For this review, take the finished solid that the model builds, in its own axes (mm). Face numbers are marked on the shaded views. Round coordinates to 2 decimals unless told otherwise and drop trailing zeros. Write each loop counter-clockwise with the first axis right and the second up, starting at its lowest first coordinate (ties: lowest second). Pieces come first, ordered by that corner, then holes. Notation, with made-up numbers: (-34.5, -38.5) - (8.5, -38.5) arc R11 ccw to (8.5, -30.5) - close; hole circle Ø8 at (45, 8.5). An arc over 180 degrees is marked (long way). Answer in a Markdown table with one row per item. Add a question column.
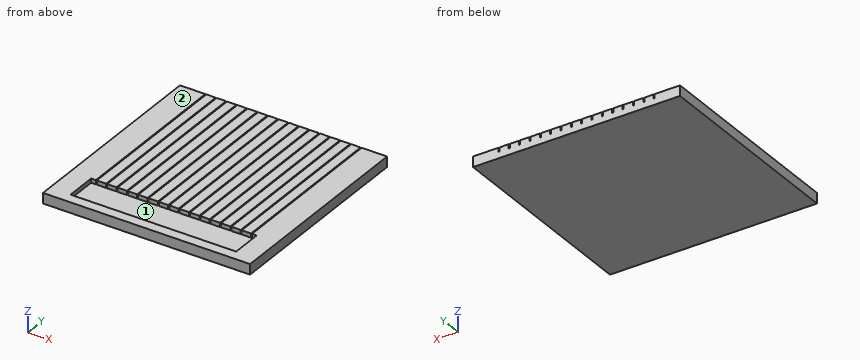
from build123d import *

# Parameters (mm, degrees)
SKETCH1_W           = 10
SKETCH1_H           = 10
BOSS_EXTRUDE1_DEPTH = 0.5
SKETCH2_W           = 8
SKETCH2_H           = 1.5
CUT_EXTRUDE1_DEPTH  = 0.2
SKETCH3_W           = 0.05
SKETCH3_H           = 8
CUT_EXTRUDE2_DEPTH  = 0.2


with BuildPart() as part:
    # Sketch1 → Boss-Extrude1 (new body)
    with BuildSketch(Plane(origin=(0, 0, 0), x_dir=(0, 1, 0), z_dir=(0, 0, 1))):
        with Locations((5, -5)):
            Rectangle(SKETCH1_W, SKETCH1_H)
    extrude(amount=BOSS_EXTRUDE1_DEPTH)

    # Sketch2 → Cut-Extrude1 (cut)
    with BuildSketch(Plane.XY.offset(0.5)):
        with Locations((5, 1.25)):
            Rectangle(SKETCH2_W, SKETCH2_H)
    extrude(amount=-CUT_EXTRUDE1_DEPTH, mode=Mode.SUBTRACT)

    # Sketch3 → Cut-Extrude2 (cut)
    with BuildSketch(Plane.XY.offset(0.5)):
        with Locations((1.25, 6)):
            Rectangle(SKETCH3_W, SKETCH3_H)
        with Locations((1.75, 6)):
            Rectangle(SKETCH3_W, SKETCH3_H)
        with Locations((2.25, 6)):
            Rectangle(SKETCH3_W, SKETCH3_H)
        with Locations((2.75, 6)):
            Rectangle(SKETCH3_W, SKETCH3_H)
        with Locations((3.25, 6)):
            Rectangle(SKETCH3_W, SKETCH3_H)
        with Locations((3.75, 6)):
            Rectangle(SKETCH3_W, SKETCH3_H)
        with Locations((4.25, 6)):
            Rectangle(SKETCH3_W, SKETCH3_H)
        with Locations((4.75, 6)):
            Rectangle(SKETCH3_W, SKETCH3_H)
        with Locations((5.25, 6)):
            Rectangle(SKETCH3_W, SKETCH3_H)
        with Locations((5.75, 6)):
            Rectangle(SKETCH3_W, SKETCH3_H)
        with Locations((6.25, 6)):
            Rectangle(SKETCH3_W, SKETCH3_H)
        with Locations((6.75, 6)):
            Rectangle(SKETCH3_W, SKETCH3_H)
        with Locations((7.25, 6)):
            Rectangle(SKETCH3_W, SKETCH3_H)
        with Locations((7.75, 6)):
            Rectangle(SKETCH3_W, SKETCH3_H)
        with Locations((8.25, 6)):
            Rectangle(SKETCH3_W, SKETCH3_H)
        with Locations((8.75, 6)):
            Rectangle(SKETCH3_W, SKETCH3_H)
    extrude(amount=-CUT_EXTRUDE2_DEPTH, mode=Mode.SUBTRACT)


solid = part.part
Q1. Add section A-A on x = 8.5. State the section outline as (y, z) points.
Q2. Add section B-B on z = 0.4. Count the separate pieces of the cut face and the enclosed holes in it, then the cut area to 3 significant figures.
Q3. Draft analysis for pull direction X (two halves, no side actions). For the marked faces 1 and 2, state which applies: released by +X, released by -X, zero draft, split by the parting line, or undercut.
Q4. To check wall thickness, follow probe 1 along Y at (x, z) = (8, 0.45); probe 2 along Z at (x, y) = (7, 0.75). State the ranges of each line that lie inside material, in increasing order.
Answer sheet:
| question | item | result |
|---|---|---|
| 1 | outline | (0, 0) - (10, 0) - (10, 0.5) - (2, 0.5) - (2, 0.3) - (0.5, 0.3) - (0.5, 0.5) - (0, 0.5) - close |
| 2 | separate pieces | 16 |
| 2 | enclosed holes | 0 |
| 2 | area | 81.6 mm² |
| 3 | face 1 | undercut |
| 3 | face 2 | zero draft |
| 4 | probe 1 | y = 0 to 0.5, 2 to 10 |
| 4 | probe 2 | z = 0 to 0.3 |
